from build123d import *

# Parameters (mm, degrees)
F1_DEPTH = 150


with BuildPart() as f1:
    # F0 (on Top) → F1 (new body)
    with BuildSketch(Plane.XY):
        with BuildLine():
            ThreePointArc((-62.509962, -36.084558), (-93.676113, 2.927788), (-62.509962, 41.940134))
            ThreePointArc((-62.509962, 41.940134), (-62.123481, 42.483344), (-62.620385, 42.927788))
            Line((-62.620385, 42.927788), (-100.961201, 42.927788))
            ThreePointArc((-100.961201, 42.927788), (-140.961201, 2.927788), (-100.961201, -37.072212))
            Line((-100.961201, -37.072212), (-62.620385, -37.072212))
            ThreePointArc((-62.620385, -37.072212), (-62.123481, -36.627767), (-62.509962, -36.084558))
        make_face()
        with BuildLine():
            ThreePointArc((-100.961201, -34.072212), (-137.961201, 2.927788), (-100.961201, 39.927788))
            Line((-100.961201, 39.927788), (-81.960385, 39.927788))
            ThreePointArc((-81.960385, 39.927788), (-80.074767, 38.594455), (-80.703306, 36.372233))
            ThreePointArc((-80.703306, 36.372233), (-96.676113, 2.927788), (-80.703306, -30.516656))
            ThreePointArc((-80.703306, -30.516656), (-80.074767, -32.738879), (-81.960385, -34.072212))
            Line((-81.960385, -34.072212), (-100.961201, -34.072212))
        make_face(mode=Mode.SUBTRACT)
    extrude(amount=F1_DEPTH)


solid = f1.part
Source: CAD feature listing. Evaluate the final solid. Frame: model axes, mm. A direction names the side the tool comes from. Give positions to 0.01 mm unless a question says otherwise; leave off trailing zeros. Loops run counter-clockwise (first coordinate to the right, second up) from the corner with the lowest first, then second, coordinate; pieces in that order, holes last. Notation, with made-up numbers: (26.5, 2.5) -> (66.5, 2.5) arc R20 cw to (66.5, 11.5) -> close; hole circle Ø5 at (4.25, 10). An arc over 180 degrees is marked (long way). Use a Markdown table: item, result. Add a question column.
1) Line query: line 1 along Y through (x, z) = (-97.5, 113.5); line 2 along Y through (x, z) = (-82, 102); line 3 along Y through (x, z) = (-69, 81). Output: solid intervals per line, ascending. Write a range as [from, to].
2) Section query B-B, the plane y = 7.5. Return the cut outline in (x, z), then the cut area to 3 significant figures.
3) Section query C-C, the plane z = 53.5. Return the cut outline in (x, y), then the cut area to 3 significant figures.
4) Section query A-A, the plane x = -99. Return the cut outline in (y, z), then the cut area to 3 significant figures.
5) First-contact query: pin 1 (3 mm diameter, centred on x = -104, z = 25, fed in from +Y); pin 2 (2 mm diameter, centred on y = 5.5, z = 63.5, fed in from +X); pin 3 (1.5 mm diameter, centred on x = -116.5, z = 67.5, fed in from -Y). Flat tips, straight axial feed; report the tip coordinate or a pass-through.
6) Pull-direction query (Y, two-part tool) for faces 1 (the face through (-96, 3, 0)), 2 (the face through (-82, 42.928, 74)), 3 (the face through (-91, -34.072, 74)), 4 (the face through (-82, -37.072, 74)); classes: +Y half, -Y half, draft (parallel to the pull), parting line (faces both ways), or undercut.
7) Reachability of faces 5 (the face through (-140.95, 3.81, 73.95)), 6 (the face through (-80.064, -32.706, 73.95)) from +Z, -Z, +X, -X, +Y, -Y: full face, straight path, thin tool, end or side. Return the list, or none.
Numbers:
| question | item | result |
|---|---|---|
| 1 | line 1 | y = [-37.07, -34.07], [39.93, 42.93] |
| 1 | line 2 | y = [-37.07, -34.07], [-29.43, -25.32], [31.17, 35.28], [39.93, 42.93] |
| 1 | line 3 | y = [-37.07, -34.02], [39.88, 42.93] |
| 2 | outline | (-140.7, 0) -> (-137.68, 0) -> (-137.68, 150) -> (-140.7, 150) -> close; (-96.43, 0) -> (-93.41, 0) -> (-93.41, 150) -> (-96.43, 150) -> close |
| 2 | area | 906 mm2 |
| 3 | outline | (-100.96, -37.07) -> (-62.62, -37.07) arc R0.5 ccw to (-62.51, -36.08) arc R40 cw to (-62.51, 41.94) arc R0.5 ccw to (-62.62, 42.93) -> (-100.96, 42.93) arc R40 ccw to start; hole (-100.96, -34.07) -> (-81.96, -34.07) arc R2 ccw to (-80.7, -30.52) arc R43 cw to (-80.7, 36.37) arc R2 ccw to (-81.96, 39.93) -> (-100.96, 39.93) arc R37 ccw to start |
| 3 | area | 869 mm2 |
| 4 | outline | (-37.07, 0) -> (-34.07, 0) -> (-34.07, 150) -> (-37.07, 150) -> close; (39.93, 0) -> (42.93, 0) -> (42.93, 150) -> (39.93, 150) -> close |
| 4 | area | 900 mm2 |
| 5 | pin 1 | stops at y = 42.9 |
| 5 | pin 2 | stops at x = -93.52 |
| 5 | pin 3 | stops at y = -34.24 |
| 6 | face 1 | draft |
| 6 | face 2 | +Y half |
| 6 | face 3 | undercut |
| 6 | face 4 | -Y half |
| 7 | face 5 | +Z, -Z, -X |
| 7 | face 6 | +Z, -Z |
